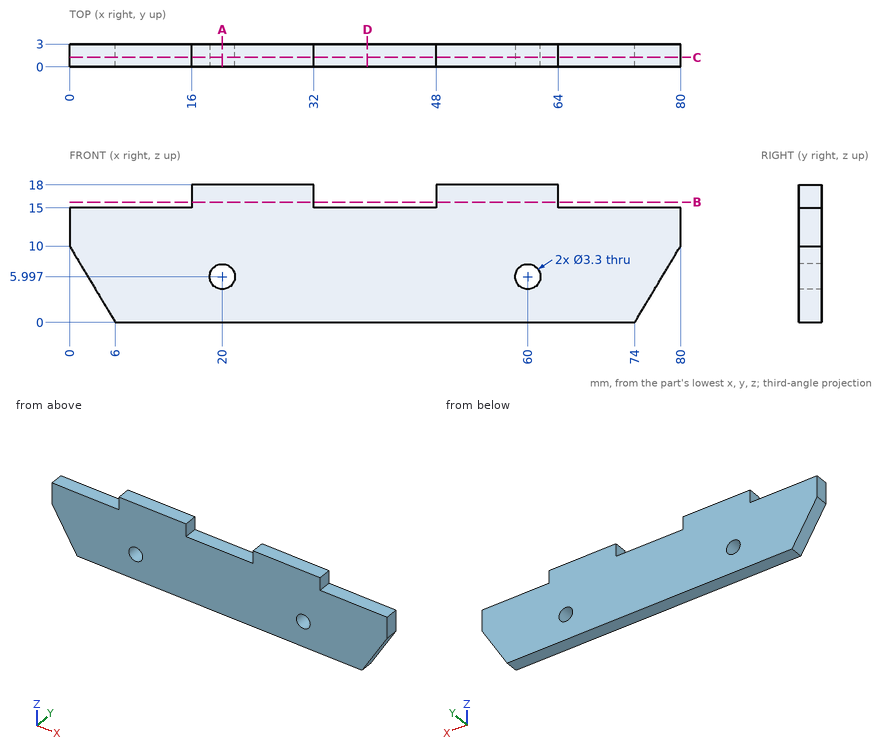
Source: three-view drawing plus pictorial views. Frame: mm from the lowest corner of the part. Coordinates: 2 decimals unless noted, no trailing zeros. Loops run counter-clockwise (first coordinate to the right, second up) from the corner with the lowest first, then second, coordinate; pieces in that order, holes last. Notation, with made-up numbers: (78, 22.5) -> (98, 22.5) arc R7 cw to (98, 26.5) -> close; hole circle Ø2 at (30, -1.5). An arc over 180 degrees is marked (long way). Write each question's results on one line, items separated by ' | '. Start each with the question number.
Q1. Ray query, line 1 (Z direction, x = 20, y = 1.7); line 2 (X direction, y = 1.65, z = 15.5); line 3 (X direction, y = 2.6, z = 5.25). Return the intervals inside material, ascending. Write a range as from..to.
Q2. Section A-A, the plane x = 20. Return the cut outline in (y, z).
Q3. Section C-C, the plane y = 1.25. Return the cut outline in (x, z), plus the area to 3 significant figures.
Q4. Pin query (flat end, axial travel): pin 1 (0.9 mm diameter, centred on x = 43.5, y = 1, fed in from +Z); pin 2 (1.5 mm diameter, centred on y = 1, z = 17, fed in from +X); pin 3 (2.5 mm diameter, centred on x = 60, z = 6, fed in from -Y). Return the tip coordinate at first contact, or that it passes through.
Q5. Section D-D, the plane x = 39. Return the cut outline in (y, z), plus the area to 3 significant figures.
Q6. Section B-B, the plane z = 15.75. Return the cut outline in (x, y).
Found:
1) line 1: 0..4.35, 7.65..18 | line 2: 16..32, 48..64 | line 3: 2.85..18.53, 21.47..58.53, 61.47..77.15
2) outline: (0, 0) -> (3, 0) -> (3, 4.35) -> (0, 4.35) -> close; (0, 7.65) -> (3, 7.65) -> (3, 18) -> (0, 18) -> close
3) outline: (0, 10) -> (6, 0) -> (74, 0) -> (80, 10) -> (80, 15) -> (64, 15) -> (64, 18) -> (48, 18) -> (48, 15) -> (32, 15) -> (32, 18) -> (16, 18) -> (16, 15) -> (0, 15) -> close; hole circle Ø3.3 at (20, 6); hole circle Ø3.3 at (60, 6) | area: 1,220 mm2
4) pin 1: z = 15 | pin 2: x = 64 | pin 3: through
5) outline: (0, 0) -> (3, 0) -> (3, 15) -> (0, 15) -> close | area: 45.0 mm2
6) outline: (16, 0) -> (32, 0) -> (32, 3) -> (16, 3) -> close; (48, 0) -> (64, 0) -> (64, 3) -> (48, 3) -> close
